For this review, take the finished solid that the model builds, in its own axes (mm). Face numbers are marked on the shaded views. A direction names the side the tool comes from. Give positions to 0.01 mm unless a question says otherwise; leave off trailing zeros. Loops run counter-clockwise (first coordinate to the right, second up) from the corner with the lowest first, then second, coordinate; pieces in that order, holes last. Notation, with made-up numbers: (31, 74) - (61, 74) arc R11 ccw to (61, 87) - close; hole circle Ø7 at (87, -37.75). An arc over 180 degrees is marked (long way). Answer in a Markdown table with one row per item.
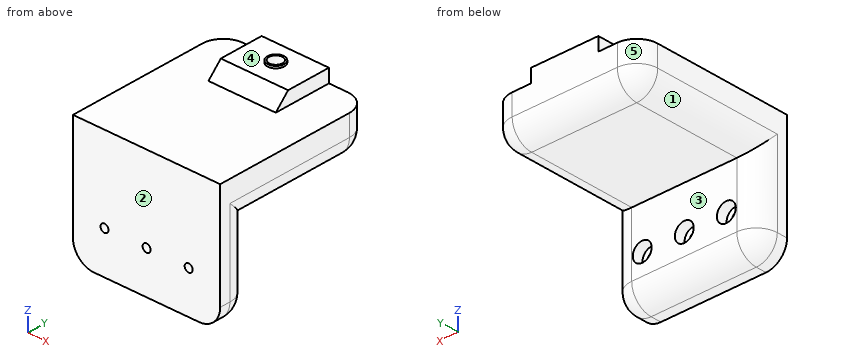
```python
from build123d import *

# Parameters (mm, degrees)
SKETCH1_W           = 70
SKETCH1_H           = 60
BOSS_EXTRUDE1_DEPTH = 15
SKETCH2_W           = 70
SKETCH2_H           = 20
BOSS_EXTRUDE2_DEPTH = 61.5
SKETCH3_R           = 3.2
CUT_EXTRUDE1_DEPTH  = 10
SKETCH5_R           = 1.9
CUT_EXTRUDE2_DEPTH  = 111.825312993
SKETCH6_R           = 4.5
CUT_EXTRUDE3_DEPTH  = 5
FILLET1_R           = 10
BOSS_EXTRUDE3_START = 6.35
SKETCH7_W           = 32
SKETCH7_H           = 20
SKETCH7_R           = 3.2
BOSS_EXTRUDE3_DEPTH = 6.35
CHAMFER1_SIZE       = 7.35
BOSS_EXTRUDE4_START = 1
SKETCH8_R           = 4
SKETCH8_R_2         = 3.2
BOSS_EXTRUDE4_DEPTH = 1


with BuildPart() as part:
    # Sketch1 → Boss-Extrude1 (new body)
    with BuildSketch(Plane(origin=(0, 0, 0), x_dir=(1, 0, 0), z_dir=(0, 1, 0))):
        with Locations((35, 30)):
            Rectangle(SKETCH1_W, SKETCH1_H)
    extrude(amount=BOSS_EXTRUDE1_DEPTH)

    # Sketch2 → Boss-Extrude2 (add)
    with BuildSketch(Plane(origin=(0, 15, 0), x_dir=(1, 0, 0), z_dir=(0, 1, 0))):
        with Locations((35, 10)):
            Rectangle(SKETCH2_W, SKETCH2_H)
    extrude(amount=BOSS_EXTRUDE2_DEPTH)

    # Sketch3 → Cut-Extrude1 (cut)
    with BuildSketch(Plane.XY):
        with Locations((35, 66.5)):
            Circle(SKETCH3_R)
    extrude(amount=-CUT_EXTRUDE1_DEPTH, mode=Mode.SUBTRACT)

    # Sketch5 → Cut-Extrude2 (cut, through all)
    with BuildSketch(Plane(origin=(0, 15, 0), x_dir=(1, 0, 0), z_dir=(0, 1, 0))):
        with Locations(Location((15, 40, 0), (0, 0, 270))):
            Circle(SKETCH5_R)
        with Locations(Location((35, 40, 0), (0, 0, 270))):
            Circle(SKETCH5_R)
        with Locations(Location((55, 40, 0), (0, 0, 270))):
            Circle(SKETCH5_R)
    extrude(amount=-CUT_EXTRUDE2_DEPTH, mode=Mode.SUBTRACT)

    # Sketch6 → Cut-Extrude3 (cut)
    with BuildSketch(Plane(origin=(0, 15, 0), x_dir=(1, 0, 0), z_dir=(0, 1, 0))):
        with Locations(Location((15, 40, 0), (0, 0, 270))):
            Circle(SKETCH6_R)
        with Locations(Location((35, 40, 0), (0, 0, 270))):
            Circle(SKETCH6_R)
        with Locations(Location((55, 40, 0), (0, 0, 270))):
            Circle(SKETCH6_R)
    extrude(amount=-CUT_EXTRUDE3_DEPTH, mode=Mode.SUBTRACT)

    # Fillet1
    fillet1_edges = [part.edges().sort_by_distance(p)[0] for p in [
        (70, 15, -40),
        (0, 45.75, -20),
        (35, 15, -60),
        (70, 45.75, -20),
        (0, 76.5, -10),
        (70, 76.5, -10),
        (35, 76.5, -20),
        (0, 15, -40),
        (0, 7.5, -60),
        (70, 7.5, -60),
    ]]
    fillet(fillet1_edges, radius=FILLET1_R)

    # Sketch7 → Boss-Extrude3 (add)
    with BuildSketch(Plane.XY.offset(BOSS_EXTRUDE3_START)):
        with Locations((35, 66.5)):
            Rectangle(SKETCH7_W, SKETCH7_H)
        with Locations((35, 66.5)):
            Circle(SKETCH7_R, mode=Mode.SUBTRACT)
    extrude(amount=-BOSS_EXTRUDE3_DEPTH)

    # Chamfer1
    # the kernel refuses this chamfer: 7.35 mm, written as the material it adds along each edge
    with BuildSketch(Plane(origin=(51, 56.5, 0), x_dir=(0, -0.9996219169112966, -0.027495876610586365), z_dir=(-1, 0, 0))) as chamfer1_piece_1_section:
        Polygon((CHAMFER1_SIZE * 0.999621916911, CHAMFER1_SIZE * 0.0274958766106), (-CHAMFER1_SIZE * 0.0274958766106, CHAMFER1_SIZE * 0.999621916911), (0, 0), align=None)
    chamfer1_piece_1 = extrude(amount=32, mode=Mode.PRIVATE)
    chamfer1_piece_1 = split(chamfer1_piece_1, bisect_by=Plane(origin=(35, 54.008386108, 6.35), z_dir=(0, 0, -1)), keep=Keep.TOP, mode=Mode.PRIVATE)
    add(chamfer1_piece_1)

    # Sketch8 → Boss-Extrude4 (add)
    with BuildSketch(Plane.XY.offset(6.35).offset(BOSS_EXTRUDE4_START)):
        with Locations((35, 66.5)):
            Circle(SKETCH8_R)
        with Locations((35, 66.5)):
            Circle(SKETCH8_R_2, mode=Mode.SUBTRACT)
    extrude(amount=-BOSS_EXTRUDE4_DEPTH)


solid = part.part
```
1. For the marked faces 1, 2, 3, 4 and 5, list the 3-axis set-ups (+Z, -Z, +X, -X, +Y, -Y) from which the entire face can be reached by the end or side of a thin tool; tool diameter is ignored.
Values:
| item | result |
|---|---|
| face 1 | -Z, -X, +Y |
| face 2 | +Z, -Z, +X, -X, -Y |
| face 3 | -Z, +X, -X, +Y |
| face 4 | +Z |
| face 5 | +Z, -Z, -X, +Y |
2. We need section A-A, the plane z = -40. Count the separate pieces of the cut face and the enclosed holes in it, and give its area (3 significant figures).
Values:
| item | result |
|---|---|
| separate pieces | 4 |
| enclosed holes | 0 |
| area | 758 mm^2 |
3. We need section B-B, the plane x = 55. Give the boundary of the cut face in (y, z).
Values:
| item | result |
|---|---|
| outline | (0, -60) - (5, -60) arc R10 ccw to (15, -50) - (15, -44.5) - (10, -44.5) - (10, -41.9) - (0, -41.9) - close; (0, -38.1) - (10, -38.1) - (10, -35.5) - (15, -35.5) - (15, -20) - (66.5, -20) arc R10 ccw to (76.5, -10) - (76.5, 0) - (0, 0) - close |
4. We need section C-C, the plane y = 61. Give the boundary of the cut face in (x, z).
Values:
| item | result |
|---|---|
| outline | (0, -10) arc R10 ccw to (10, -20) - (60, -20) arc R10 ccw to (70, -10) - (70, 0) - (51, 0) - (51, 6.35) - (19, 6.35) - (19, 0) - (0, 0) - close |
5. Clearance check with flat-ended pins moving along their axes: pin 1 (10.5 mm diameter, centred on x = 15, z = -40, fed in from +Y); pin 2 (5 mm diameter, centred on x = 35, y = 18, fed in from -Z); pin 3 (2 mm diameter, centred on x = 7.5, y = 17, fed in from -Z). State where each tip first meets the part, or that it passes through.
Values:
| item | result |
|---|---|
| pin 1 | stops at y = 15 |
| pin 2 | stops at z = -20 |
| pin 3 | stops at z = -19.89 |
6. Wall thickness on line 1 (X direction, y = 4, z = -40); line 2 (Y direction, x = 35, z = -3); line 3 (Z direction, x = 56, y = 61): over which ranges is each line inside the solid? List them lowest first. Write a range as [from, to].
Values:
| item | result |
|---|---|
| line 1 | x = [0, 13.1], [16.9, 33.1], [36.9, 53.1], [56.9, 70] |
| line 2 | y = [0, 63.3], [69.7, 76.5] |
| line 3 | z = [-20, 0] |
7. We need section D-D, the plane y = 12.5. Give the boundary of the cut face in (x, z).
Values:
| item | result |
|---|---|
| outline | (0, -10) arc R10 ccw to (3.39, -17.5) - (3.39, -50) arc R6.61 ccw to (10, -56.61) - (60, -56.61) arc R6.61 ccw to (66.61, -50) - (66.61, -17.5) arc R10 ccw to (70, -10) - (70, 0) - (0, 0) - close; hole circle Ø9 at (15, -40); hole circle Ø9 at (35, -40); hole circle Ø9 at (55, -40) |
